Autodesk Inventor part; units mm, degrees
ref_plane "Work Plane1" through (7.9977, -5.9583, -3) normal (0, 0, 1) x (1, 0, 0)
ref_plane "YZ Plane" through (0, 0, 0) normal (1, 0, 0) x (0, 1, 0)
ref_plane "XZ Plane" through (0, 0, 0) normal (0, 1, 0) x (-1, 0, 0)
sketch "Sketch1" plane through (0, 0, 0) normal (0, 0, 1) x (1, 0, 0)
  circle A0 centre (-4.0482, 0) radius 1.45
  circle A1 centre (4.0482, 0) radius 1.45
  line L0 (-8, 3.9518) -> (-8, -3.9518)
  line L1 (-8, -3.9518) -> (8, -3.9518)
  line L2 (8, -3.9518) -> (8, 3.9518)
  line L3 (8, 3.9518) -> (-8, 3.9518)
  line L4 (8.2, 4.1518) -> (8.2, -4.1518)
  line L5 (8.2, -4.1518) -> (-8.2, -4.1518)
  line L6 (-8.2, -4.1518) -> (-8.2, 4.1518)
  line L7 (-8.2, 4.1518) -> (8.2, 4.1518)
  point P0 (0, 0)
  dimension "d0" = 0.2
extrude "Extrusion1" add sketch "Sketch1" along normal blind 2 contours L3 L2 L1 L0 | L4 L5 L6 L7
sketch "Sketch2" plane through (0, 0, 2) normal (0, 0, 1) x (1, 0, 0)
  line L0 (8.2, -4.1518) -> (8.2, 4.1518)
  line L1 (8.2, 4.1518) -> (-8.2, 4.1518)
  line L2 (-8.2, 4.1518) -> (-8.2, -4.1518)
  line L3 (-8.2, -4.1518) -> (8.2, -4.1518)
  line L4 (9.7, 5.6518) -> (9.7, -5.6518)
  line L5 (9.7, -5.6518) -> (-9.7, -5.6518)
  line L6 (-9.7, -5.6518) -> (-9.7, 5.6518)
  line L7 (-9.7, 5.6518) -> (9.7, 5.6518)
  point P0 (0, 0)
  dimension "d3" = 1.5
ref_plane "Work Plane1" through (7.9977, -5.9583, -3) normal (0, 0, 1) x (1, 0, 0)
extrude "Extrusion2" add sketch "Sketch2" against normal up to surface (5 mm away)
sketch "Sketch3" plane through (-9.7, 5.6518, 2) normal (0, 1, 0) x (1, 0, 0)
  line L0 (0, 0) -> (0, 5)
  line L1 (0, 0) -> (0, -18)
  circle A0 centre (0, -18) radius 18
  circle A1 centre (0, -18) radius 23
  line L2 (0, -18) -> (-16.2635, -1.7365)
  line L3 (0, -18) -> (23, -18) construction
  point P0 (9.7, 2)
  point P1 (-12.7279, -5.2721)
  dimension "d6" = 18
  dimension "d7" = 135
extrude "Extrusion3" add sketch "Sketch3" against normal up to surface (11.3036 mm away) contours A0 L2 A1 L0 picked at (-13.0139, -1.2154)
sketch "Sketch5" plane through (9.7, 5.6518, 2) normal (0, 1, 0) x (1, 0, 0)
  line L0 (-35.6635, -1.7365) -> (-32.1279, -5.2721)
  line L1 (-35.6635, -1.7365) -> (-32.1279, -5.2721)
  line L2 (-32.1279, -5.2721) -> (-37.0777, -10.2218)
  line L3 (-37.0777, -10.2218) -> (-40.6132, -6.6863)
  line L4 (-40.6132, -6.6863) -> (-35.6635, -1.7365)
  point P0 (-9.7, 2)
  dimension "d10" = 7
extrude "Extrusion4" add sketch "Sketch5" against normal up to surface (11.3036 mm away)
sketch "Sketch6" plane through (9.7, -5.6518, -3) normal (0, -1, 0) x (1, 0, 0)
  line L0 (-37.0777, 15.2218) -> (-32.1279, 10.2721)
  arc A0 (-32.1279, 10.2721) -> (-19.4, 5) centre (-19.4, 23) ccw
  line L1 (-40.6132, 11.6863) -> (-37.0777, 15.2218)
  line L2 (-35.6635, 6.7365) -> (-40.6132, 11.6863)
  arc A1 (-35.6635, 6.7365) -> (-19.4, 0) centre (-19.4, 23) ccw
  line L3 (-19.4, 5) -> (0, 5)
  line L4 (0, 0) -> (-19.4, 0)
  line L5 (-15.1982, 5) -> (-15.1982, 3)
  line L6 (-15.1982, 5) -> (-15.1982, 0)
  point P0 (-9.7, 3)
extrude "Extrusion5" add sketch "Sketch6" along normal blind 15
sketch "Sketch7" plane through (9.7, 5.6518, 2) normal (0, 1, 0) x (1, 0, 0)
  line L0 (-32.1279, -5.2721) -> (-37.0777, -10.2218)
  line L1 (-37.0777, -10.2218) -> (-40.6132, -6.6863)
  line L2 (-40.6132, -6.6863) -> (-35.6635, -1.7365)
  arc A0 (-19.4, 5) -> (-35.6635, -1.7365) centre (-19.4, -18) ccw
  line L3 (-19.4, 5) -> (-15.1982, 5)
  line L4 (-15.1982, 5) -> (-15.1982, 0)
  line L5 (-15.1982, 0) -> (-19.4, 0)
  arc A1 (-19.4, 0) -> (-32.1279, -5.2721) centre (-19.4, -18) ccw
  point P0 (-9.7, 2)
extrude "Extrusion6" add sketch "Sketch7" along normal blind 15
sketch "Sketch8" plane through (-5.4982, 5.6518, 2) normal (1, 0, 0) x (0, 0, -1)
  line L0 (-43.306, 51.1457) -> (8.0398, -0.2)
  line L1 (8.0154, -11.1036) -> (-43.306, -62.425)
  line L2 (-44.7202, 49.7315) -> (6.6255, -1.6142)
  line L3 (6.6012, -9.6894) -> (-44.7202, -61.0108)
  line L4 (5, 0) -> (5, 15)
  line L5 (-10.2218, 15) -> (-5.2721, 15)
  line L6 (-5.2721, 15) -> (0, 15)
  line L7 (0, 15) -> (5, 15)
  line L8 (5, -11.3036) -> (5, -26.3036)
  line L9 (5, -26.3036) -> (0, -26.3036)
  line L10 (0, -26.3036) -> (-5.2721, -26.3036)
  line L11 (-5.2721, -26.3036) -> (-10.2218, -26.3036)
  line L12 (0, -11.3036) -> (5, -11.3036)
  point P0 (2, -5.6518)
  point P1 (-9.9887, 15)
  point P2 (5, 0.0113)
  point P3 (4.987, -11.3036)
  point P4 (-10.013, -26.3036)
  dimension "d17" = 2
  dimension "d18" = 2
extrude "Extrusion7" cut sketch "Sketch8" against normal through all
properties part number "KickerFoot_3DPrint"
Geometry check sheet. Reference: the model listing, model coordinates, mm. A direction names the side the tool comes from. Give positions to 0.01 mm unless a question says otherwise; leave off trailing zeros. Write each loop counter-clockwise with the first axis right and the second up, starting at its lowest first coordinate (ties: lowest second). Pieces come first, ordered by that corner, then holes. Notation, with made-up numbers: M 41,-3.75 L 65,-3.75 A18 cw 65,11.25 Z; hole C 35,-29 d2. An arc over 180 degrees is marked long. One line per question, with ' | ' between items.
1. Cross-section at D-D (z = 5.75). Enter the section's corners in (x, y), plus the area to 3 significant figures.
Ans:
outline: M -27.98,-14.39 L -20.7,-14.39 L -20.7,5.65 L -20.7,14.41 L -27.98,14.41 Z | area: 210 mm2
2. Cross-section at B-B (y = 0). Enter the section's corners in (x, z).
Ans:
outline: M -30.91,8.69 L -25.96,3.74 A23 ccw -9.7,-3 L -8.2,-3 L -8.2,0 L -5.5,0 L -5.5,2 L -9.7,2 A18 cw -22.43,7.27 L -27.38,12.22 Z; M -2.6,0 L 2.6,0 L 2.6,2 L -2.6,2 Z; M 5.5,0 L 8.2,0 L 8.2,-3 L 9.7,-3 L 9.7,2 L 5.5,2 Z
3. Cross-section at A-A (x = -4.5). Enter the section's corners in (y, z), plus the area to 3 significant figures.
Ans:
outline: M -5.65,-3 L -4.15,-3 L -4.15,0 L -1.38,0 L -1.38,2 L -5.65,2 Z; M 1.38,0 L 4.15,0 L 4.15,-3 L 5.65,-3 L 5.65,2 L 1.38,2 Z | area: 26.1 mm2
4. Set-up check for faces 5 (the face through (-17.924, -9.57, 3.988)), 6 (the face through (-5.498, 8, 0)), 7 (the face through (-5.498, -8, 0)): record each of +Z, -Z, +X, -X, +Y, -Y from which the full face is reachable in a straight line by a thin tool's end or side.
Ans:
face 5: +Z, +X, +Y, -Y | face 6: +Z, -Z, +X, +Y | face 7: +Z, -Z, +X, -Y
5. Mould release check, pull along Y, two halves, no side actions. Record for faces 1 (the face through (0, -4.152, -1)), 2 (the face through (0, 0, 0)), 3 (the face through (0, 5, -3)), 4 (the face through (-18.03, -11.38, 2.74)): released by +Y, released by -Y, zero draft, split by the parting line, or undercut.
Ans:
face 1: undercut | face 2: undercut | face 3: zero draft | face 4: released by -Y
6. Cross-section at C-C (x = 0.5). Enter the section's corners in (y, z), plus the area to 3 significant figures.
Ans:
outline: M -5.65,-3 L -4.15,-3 L -4.15,0 L 4.15,0 L 4.15,-3 L 5.65,-3 L 5.65,2 L -5.65,2 Z | area: 31.6 mm2
7. Scan lines: line 1 along Z through (x, y) = (8, 5); line 2 along Y through (x, z) = (1.5, -2.5); line 3 along X through (y, z) = (1, -1). Record each from-to range of solid material in increasing order. Write a range as from..to.
Ans:
line 1: -3..2 | line 2: -5.65..-4.15, 4.15..5.65 | line 3: -19.08..-8.2, 8.2..9.7
8. Gauge pin test, flat ends, axial feed: pin 1 (0.9 mm diameter, centred on x = -1, z = -1.5, fed in from +Y); pin 2 (1.5 mm diameter, centred on x = -17.5, z = 4, fed in from -Y); pin 3 (4 mm diameter, centred on x = -4.05, y = 0, fed in from -Z); pin 4 (3 mm diameter, centred on x = -8.5, y = 13, fed in from +Z). Record the tip position at first contact, or that the pin passes through.
Ans:
pin 1: y = 5.65 | pin 2: y = -12.79 | pin 3: z = 0 | pin 4: through
